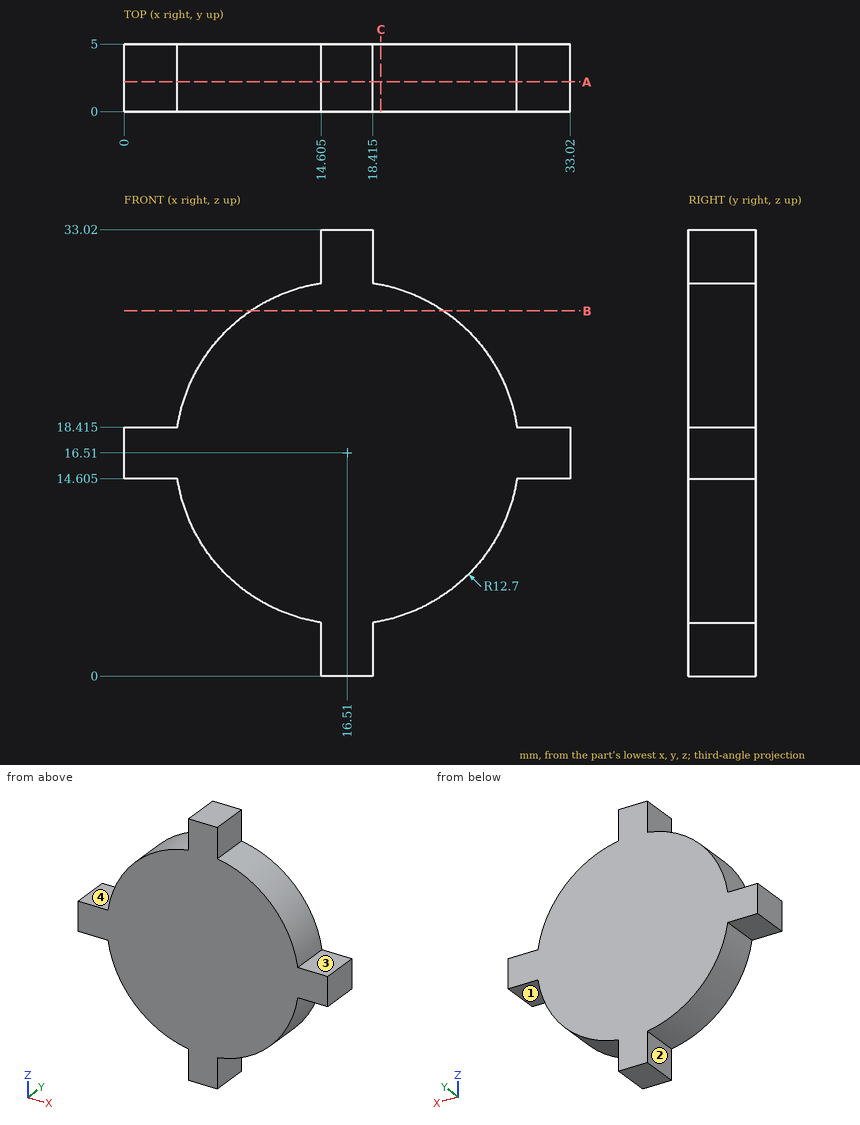
The drawing under review shows one solid part. Ordinate dimensions are in mm from its lowest x, y, z. A direction names the side the tool comes from. Coordinates: 2 decimals unless noted, no trailing zeros. Order: outer loops, then holes, each group sorted by start corner. A loop starts at its lowest first (then second) coordinate and runs counter-clockwise, first axis right, second up. Notation, with made-up numbers: M 57,52.25 L 91,52.25 A26 cw 91,88.25 Z; hole C 71.25,34 d6. An arc over 180 degrees is marked long. Use a Markdown table: item, result.
(1) Add section C-C (x = 19). Give the boundary of the cut face in (y, z), then the cut area to 3 significant figures.
Worked answers:
| item | result |
|---|---|
| outline | M 0,4.06 L 5,4.06 L 5,28.96 L 0,28.96 Z |
| area | 125 mm2 |
(2) Wall thickness on probe 1 along X at (y, z) = (3.4, 30) (3 decimals); probe 2 along Z at (x, y) = (20, 4.6): over which ranges is each line inside the solid? List them lowest first.
Worked answers:
| item | result |
|---|---|
| probe 1 | x = 14.605 to 18.415 |
| probe 2 | z = 4.3 to 28.72 |
(3) For P1, Ø1.5, axis at x = 6, z = 11.5, coming from the -Y side; P2, Ø1.5, axis at x = 23, y = 1.5, coming from the -Z side; P3, Ø1.2, axis at y = 1.5, z = 1, coming from the +X side (3 decimals); P4, Ø2, axis at x = 31.5, y = 2.5, coming from the +Z side (3 decimals), all flat-tipped, find the tip position at first contact; note any pin that passes through.
Worked answers:
| item | result |
|---|---|
| P1 | stops at y = 0 |
| P2 | stops at z = 5.18 |
| P3 | stops at x = 18.415 |
| P4 | stops at z = 18.415 |
(4) Add section A-A (y = 2.2). Give the boundary of the cut face in (x, z) (3 decimals), then the cut area to 4 significant figures.
Worked answers:
| item | result |
|---|---|
| outline | M 0,14.605 L 3.954,14.605 A12.7 ccw 14.605,3.954 L 14.605,0 L 18.415,0 L 18.415,3.954 A12.7 ccw 29.066,14.605 L 33.02,14.605 L 33.02,18.415 L 29.066,18.415 A12.7 ccw 18.415,29.066 L 18.415,33.02 L 14.605,33.02 L 14.605,29.066 A12.7 ccw 3.954,18.415 L 0,18.415 Z |
| area | 565.5 mm2 |
(5) Add section B-B (z = 27). Give the boundary of the cut face in (x, y).
Worked answers:
| item | result |
|---|---|
| outline | M 9.35,0 L 23.67,0 L 23.67,5 L 9.35,5 Z |
(6) For the marked faces 1, 2, 3 and 4, list the 3-axis set-ups (+Z, -Z, +X, -X, +Y, -Y) from which the entire face can be reached by the end or side of a thin tool; tool diameter is ignored.
Worked answers:
| item | result |
|---|---|
| face 1 | -Z, +X, +Y, -Y |
| face 2 | -Z, -X, +Y, -Y |
| face 3 | +Z, +X, +Y, -Y |
| face 4 | +Z, -X, +Y, -Y |
